from build123d import *

# Parameters (mm, degrees)
SKETCH_1_W              = 400
SKETCH_1_H              = 160
EXTRUDE_1_DEPTH         = 10
CUT_EXTRUDE_1_DEPTH     = 2.7
FILLET_1_R              = 0.13
FILLET_2_R              = 0.5
CUT_EXTRUDE_2_DEPTH     = 432.277173057
HOLE_WIZARD_M12_1_D     = 10.2
HOLE_WIZARD_M12_1_DEPTH = 15
HOLE_WIZARD_M12_1_TIP   = 3.064389157
HOLE_WIZARD_M8_1_D      = 6.8
HOLE_WIZARD_M8_1_DEPTH  = 15
HOLE_WIZARD_M8_1_TIP    = 2.042926105


with BuildPart() as part:
    # 스케치1 → 보스-돌출1 (new, symmetric)
    with BuildSketch(Plane(origin=(0, 0, 0), x_dir=(1, 0, 0), z_dir=(0, 1, 0))):
        with Locations((200, 80)):
            Rectangle(SKETCH_1_W, SKETCH_1_H)
    extrude(amount=EXTRUDE_1_DEPTH, both=True)

    # 스케치2 → 컷-돌출1 (cut)
    with BuildSketch(Plane(origin=(0, 10, 0), x_dir=(1, 0, 0), z_dir=(0, 1, 0))):
        with BuildLine():
            Line((92, 137.05), (308, 137.05))
            ThreePointArc((308, 137.05), (333.491199462, 126.491199462), (344.05, 101))
            Line((344.05, 101), (344.05, 78))
            ThreePointArc((344.05, 78), (333.491199462, 52.508800538), (308, 41.95))
            Line((308, 41.95), (92, 41.95))
            ThreePointArc((92, 41.95), (66.508800538, 52.508800538), (55.95, 78))
            Line((55.95, 78), (55.95, 101))
            ThreePointArc((55.95, 101), (66.508800538, 126.491199462), (92, 137.05))
        make_face()
        with BuildLine():
            Line((92, 132.95), (308, 132.95))
            ThreePointArc((308, 132.95), (330.592061659, 123.592061659), (339.95, 101))
            Line((339.95, 101), (339.95, 78))
            ThreePointArc((339.95, 78), (330.592061659, 55.407938341), (308, 46.05))
            Line((308, 46.05), (92, 46.05))
            ThreePointArc((92, 46.05), (69.407938341, 55.407938341), (60.05, 78))
            Line((60.05, 78), (60.05, 101))
            ThreePointArc((60.05, 101), (69.407938341, 123.592061659), (92, 132.95))
        make_face(mode=Mode.SUBTRACT)
    extrude(amount=-CUT_EXTRUDE_1_DEPTH, mode=Mode.SUBTRACT)

    # 필렛1
    fillet_1_edges = [part.edges().sort_by_distance(p)[0] for p in [
        (66.508800538, 10, -126.491199462),
        (55.95, 10, -89.5),
        (66.508800538, 10, -52.508800538),
        (200, 10, -41.95),
        (333.491199462, 10, -52.508800538),
        (344.05, 10, -89.5),
        (333.491199462, 10, -126.491199462),
        (200, 10, -137.05),
        (69.407938341, 10, -123.592061659),
        (200, 10, -132.95),
        (330.592061659, 10, -123.592061659),
        (339.95, 10, -89.5),
        (330.592061659, 10, -55.407938341),
        (200, 10, -46.05),
        (69.407938341, 10, -55.407938341),
        (60.05, 10, -89.5),
    ]]
    fillet(fillet_1_edges, radius=FILLET_1_R)

    # 필렛2
    fillet_2_edges = [part.edges().sort_by_distance(p)[0] for p in [
        (66.508800538, 7.3, -126.491199462),
        (200, 7.3, -137.05),
        (333.491199462, 7.3, -126.491199462),
        (344.05, 7.3, -89.5),
        (333.491199462, 7.3, -52.508800538),
        (200, 7.3, -41.95),
        (66.508800538, 7.3, -52.508800538),
        (55.95, 7.3, -89.5),
        (200, 7.3, -132.95),
        (69.407938341, 7.3, -123.592061659),
        (60.05, 7.3, -89.5),
        (69.407938341, 7.3, -55.407938341),
        (200, 7.3, -46.05),
        (330.592061659, 7.3, -55.407938341),
        (339.95, 7.3, -89.5),
        (330.592061659, 7.3, -123.592061659),
    ]]
    fillet(fillet_2_edges, radius=FILLET_2_R)

    # 스케치3 → 컷-돌출2 (cut, through all)
    with BuildSketch(Plane(origin=(0, 10, 0), x_dir=(1, 0, 0), z_dir=(0, 1, 0))):
        with BuildLine():
            Line((92, 118), (308, 118))
            ThreePointArc((308, 118), (315.071067812, 115.071067812), (318, 108))
            Line((318, 108), (318, 82))
            ThreePointArc((318, 82), (315.071067812, 74.928932188), (308, 72))
            Line((308, 72), (92, 72))
            ThreePointArc((92, 72), (84.928932188, 74.928932188), (82, 82))
            Line((82, 82), (82, 108))
            ThreePointArc((82, 108), (84.928932188, 115.071067812), (92, 118))
        make_face()
    extrude(amount=-CUT_EXTRUDE_2_DEPTH, mode=Mode.SUBTRACT)

    # M12 나사 구멍1
    with Locations(Plane(origin=(0, 10, 0), x_dir=(1, 0, 0), z_dir=(0, 1, 0))):
        with Locations((58, 45), (343, 45)):
            Hole(HOLE_WIZARD_M12_1_D / 2, depth=HOLE_WIZARD_M12_1_DEPTH)
            with Locations((0, 0, -(HOLE_WIZARD_M12_1_DEPTH + HOLE_WIZARD_M12_1_TIP / 2))):  # 118° drill point
                Cone(0, HOLE_WIZARD_M12_1_D / 2, HOLE_WIZARD_M12_1_TIP, mode=Mode.SUBTRACT)

    # M8 나사 구멍1
    with Locations(Plane(origin=(0, 10, 0), x_dir=(1, 0, 0), z_dir=(0, 1, 0))):
        with Locations((45, 128), (45, 45), (355, 128), (355, 45)):
            Hole(HOLE_WIZARD_M8_1_D / 2, depth=HOLE_WIZARD_M8_1_DEPTH)
            with Locations((0, 0, -(HOLE_WIZARD_M8_1_DEPTH + HOLE_WIZARD_M8_1_TIP / 2))):  # 118° drill point
                Cone(0, HOLE_WIZARD_M8_1_D / 2, HOLE_WIZARD_M8_1_TIP, mode=Mode.SUBTRACT)


solid = part.part
Design review of the part built by this model. Coordinates are the model's own, in mm. A direction names the side the tool comes from. Give positions to 0.01 mm unless a question says otherwise; leave off trailing zeros. Loops run counter-clockwise (first coordinate to the right, second up) from the corner with the lowest first, then second, coordinate; pieces in that order, holes last. Notation, with made-up numbers: (24.25, 22) - (46.25, 22) arc R33 ccw to (46.25, 58) - close; hole circle Ø2 at (-13, 66). An arc over 180 degrees is marked (long way). Use CSV: the item, a comma, the result in double quotes. Start each with the question number.
1. Draft analysis for pull direction X (two halves, no side actions). For faces 1 (the flat face through (197, 0, 0)), 2 (the conical face through (342.115, -7.532, -45.039)), state which applies: released by +X, released by -X, zero draft, split by the parting line, or undercut.
2. Machinability: for faces 3 (the cylindrical face through (66.79, 8.85, -52.23)), 4 (the flat face through (197, 0, -160)), 5 (the flat face through (318, 0, -95)), which of the approach directions +Z, -Z, +X, -X, +Y, -Y give a long, thin tool a straight path to every point of the face, cutting with its end or side? Answer none if there is none.
3. Wall thickness on L1, parallel to Z at x = 355, y = 0; L2, parallel to X at y = 6, z = -45; L3, parallel to Z at x = 150.5, y = 5.5: over which ranges is each line inside the solid? List them lowest first.
4. Add section C-C (y = 3.5). State the section outline as (x, z) points.
5. Add section A-A (x = 203). State the section outline as (y, z) points.
6. Add section B-B (z = -94). State the section outline as (x, y) points.
Results found:
1,face 1,"zero draft"
1,face 2,"undercut"
2,face 3,"+Y"
2,face 4,"-Z, +X, -X, +Y, -Y"
2,face 5,"+Y, -Y"
3,L1,"z = -160 to -131.4, -124.6 to -48.4, -41.6 to 0"
3,L2,"x = 0 to 41.6, 48.4 to 52.9, 63.1 to 337.9, 348.1 to 351.6, 358.4 to 400"
3,L3,"z = -160 to -118, -72 to 0"
4,outline,"(0, -160) - (400, -160) - (400, 0) - (0, 0) - close; hole circle Ø6.8 at (45, -128); hole circle Ø6.8 at (45, -45); hole circle Ø10.2 at (58, -45); hole (82, -108) arc R10 ccw to (92, -118) - (308, -118) arc R10 ccw to (318, -108) - (318, -82) arc R10 ccw to (308, -72) - (92, -72) arc R10 ccw to (82, -82) - close; hole circle Ø10.2 at (343, -45); hole circle Ø6.8 at (355, -128); hole circle Ø6.8 at (355, -45)"
5,outline,"(-10, -160) - (10, -160) - (10, -137.18) arc R0.13 ccw to (9.87, -137.05) - (7.8, -137.05) arc R0.5 cw to (7.3, -136.55) - (7.3, -133.45) arc R0.5 cw to (7.8, -132.95) - (9.87, -132.95) arc R0.13 ccw to (10, -132.82) - (10, -118) - (-10, -118) - close; (-10, -72) - (10, -72) - (10, -46.18) arc R0.13 ccw to (9.87, -46.05) - (7.8, -46.05) arc R0.5 cw to (7.3, -45.55) - (7.3, -42.45) arc R0.5 cw to (7.8, -41.95) - (9.87, -41.95) arc R0.13 ccw to (10, -41.82) - (10, 0) - (-10, 0) - close"
6,outline,"(0, -10) - (82, -10) - (82, 10) - (60.18, 10) arc R0.13 ccw to (60.05, 9.87) - (60.05, 7.8) arc R0.5 cw to (59.55, 7.3) - (56.45, 7.3) arc R0.5 cw to (55.95, 7.8) - (55.95, 9.87) arc R0.13 ccw to (55.82, 10) - (0, 10) - close; (318, -10) - (400, -10) - (400, 10) - (344.18, 10) arc R0.13 ccw to (344.05, 9.87) - (344.05, 7.8) arc R0.5 cw to (343.55, 7.3) - (340.45, 7.3) arc R0.5 cw to (339.95, 7.8) - (339.95, 9.87) arc R0.13 ccw to (339.82, 10) - (318, 10) - close"
